from build123d import *

# Parameters (mm, degrees)
SKETCH1_W               = 15
SKETCH1_H               = 40
BOSS_EXTRUDE1_DEPTH     = 130
SKETCH2_W               = 15
SKETCH2_H               = 117.5
CUT_EXTRUDE1_DEPTH      = 30
CUT_EXTRUDE2_DEPTH      = 133.594306062
CUT_EXTRUDE2_DEPTH_BACK = 133.594306062
SKETCH3_R               = 1.5
SKETCH4_W               = 15
SKETCH4_H               = 6.25
BOSS_EXTRUDE2_DEPTH     = 10
SKETCH5_W               = 15
SKETCH5_H               = 9.54020797
BOSS_EXTRUDE3_DEPTH     = 10
FILLET1_R               = 10
SKETCH7_W               = 15
SKETCH7_H               = 6.25
CUT_EXTRUDE3_DEPTH      = 10


with BuildPart() as part:
    # Sketch1 → Boss-Extrude1 (new body)
    with BuildSketch(Plane.XY):
        with Locations((0, 5)):
            Rectangle(SKETCH1_W, SKETCH1_H)
    extrude(amount=BOSS_EXTRUDE1_DEPTH)

    # Sketch2 → Cut-Extrude1 (cut)
    with BuildSketch(Plane(origin=(0, 25, 0), x_dir=(1, 0, 0), z_dir=(0, 1, 0))):
        with Locations((0, -65)):
            Rectangle(SKETCH2_W, SKETCH2_H)
    extrude(amount=-CUT_EXTRUDE1_DEPTH, mode=Mode.SUBTRACT)

    # Sketch3 → Cut-Extrude2 (cut, two sides: drawn at the far end of the back side and taken through both)
    with BuildSketch(Plane(origin=(0, 0, 0), x_dir=(-1, 0, 0), z_dir=(0, 0, -1)).offset(-CUT_EXTRUDE2_DEPTH_BACK)):
        with Locations((0.28935703, 16.716588701)):
            Circle(SKETCH3_R)
        with Locations((0.28935703, -3.283411299)):
            Circle(SKETCH3_R)
    extrude(amount=CUT_EXTRUDE2_DEPTH + CUT_EXTRUDE2_DEPTH_BACK, mode=Mode.SUBTRACT)

    # Sketch4 → Boss-Extrude2 (add)
    with BuildSketch(Plane(origin=(0, 25, 0), x_dir=(1, 0, 0), z_dir=(0, 1, 0))):
        with Locations((0, -3.125)):
            Rectangle(SKETCH4_W, SKETCH4_H)
        with Locations((0, -126.875)):
            Rectangle(SKETCH4_W, SKETCH4_H)
    extrude(amount=BOSS_EXTRUDE2_DEPTH)

    # Sketch5 → Boss-Extrude3 (add)
    with BuildSketch(Plane(origin=(0, 0, 123.75), x_dir=(-1, 0, 0), z_dir=(0, 0, -1))):
        with Locations((0, 30.229896015)):
            Rectangle(SKETCH5_W, SKETCH5_H)
    extrude(amount=BOSS_EXTRUDE3_DEPTH)

    # Fillet1
    fillet1_edges = [part.edges().sort_by_distance(p)[0] for p in [
        (7.5, 35, 3.125),
        (7.5, 35, 121.875),
    ]]
    fillet(fillet1_edges, radius=FILLET1_R)

    # Sketch7 → Cut-Extrude3 (cut)
    with BuildSketch(Plane(origin=(0, 35, 0), x_dir=(1, 0, 0), z_dir=(0, 1, 0))):
        with Locations((0, -3.125)):
            Rectangle(SKETCH7_W, SKETCH7_H)
    extrude(amount=-CUT_EXTRUDE3_DEPTH, mode=Mode.SUBTRACT)


solid = part.part
Source: CAD feature listing. Evaluate the final solid. Frame: model axes, mm. A direction names the side the tool comes from. Give positions to 0.01 mm unless a question says otherwise; leave off trailing zeros. Write each loop counter-clockwise with the first axis right and the second up, starting at its lowest first coordinate (ties: lowest second). Pieces come first, ordered by that corner, then holes. Notation, with made-up numbers: (15.25, 26.25) - (58.25, 26.25) arc R14 ccw to (58.25, 35.25) - close; hole circle Ø1 at (86, 57). An arc over 180 degrees is marked (long way). Write item = value, one per line. Start each with the question number.
Q1. Cut plane A-A, the plane y = 6. Return loops of the section in (x, z).
Q2. Cut plane C-C, the plane z = 81. Return loops of the section in (x, y).
Q3. Draft query along X for faces 1 (the cylindrical face through (-0.982, -4.614, 126.919)), 2 (the flat face through (7.5, -7, 65)), 3 (the flat face through (0, 10, 130)). Return one class per face: +X half, -X half, draft (parallel to the pull), parting line (faces both ways), or undercut.
Q4. Material intervals for probe 1 along Z at (x, y) = (-0.75, -1.5); probe 2 along Y at (x, z) = (-5.5, 116); probe 3 along Y at (x, z) = (6.5, 112), sorted ascending.
Q5. Pin query (flat end, axial travel): pin 1 Ø1.8 at (x, y) = (-0.29, 16.72) entering from +Z; pin 2 Ø7.5 at (x, y) = (1.5, 29.5) entering from -Z; pin 3 Ø5 at (x, z) = (2, 2.5) entering from +Y; pin 4 Ø2 at (x, z) = (6, 35) entering from +Y. Return the tip coordinate at first contact, or that it passes through.
Q6. Cut plane D-D, the plane x = -5.5. Return loops of the section in (y, z).
Q7. Reachability of faces 4 (the flat face through (0, 25.46, 119)), 5 (the flat face through (-5, 35, 122)), 6 (the flat face through (0, 10, 123.75)), 7 (the flat face through (0, 10, 6.25)), 8 (the flat face through (-2, 30, 113.75)) from +Z, -Z, +X, -X, +Y, -Y: full face, straight path, thin tool, end or side. Return the list, or none.
Q8. Cut plane B-B, the plane x = 3.5. Return loops of the section in (y, z), then the cut area to 3 significant figures.
Computed values:
q1.outline = (-7.5, 0) - (7.5, 0) - (7.5, 6.25) - (-7.5, 6.25) - close; (-7.5, 123.75) - (7.5, 123.75) - (7.5, 130) - (-7.5, 130) - close
q2.outline = (-7.5, -15) - (7.5, -15) - (7.5, -5) - (-7.5, -5) - close
q3.face_1 = undercut
q3.face_2 = +X half
q3.face_3 = draft
q4.probe_1 = 0 to 6.25, 123.75 to 130
q4.probe_2 = -15 to -5, 25.46 to 35
q4.probe_3 = -15 to -5
q5.pin_1 = through
q5.pin_2 = 113.75
q5.pin_3 = 25
q5.pin_4 = -5
q6.outline = (-15, 0) - (25, 0) - (25, 6.25) - (-5, 6.25) - (-5, 123.75) - (25.46, 123.75) - (25.46, 113.75) - (35, 113.75) - (35, 130) - (-15, 130) - close
q7.face_4 = -Z, +X, -X
q7.face_5 = +Z, -Z, +X, -X, +Y
q7.face_6 = +X, -X
q7.face_7 = +X, -X, +Y
q7.face_8 = -Z, +X, -X, +Y
q8.outline = (-15, 0) - (25, 0) - (25, 6.25) - (-5, 6.25) - (-5, 123.75) - (25.46, 123.75) - (25.46, 113.75) - (33, 113.75) - (33, 130) - (-15, 130) - close
q8.area = 1,800 mm²
